Geometry check sheet. Reference: the model listing, model coordinates, mm. Face numbers are marked on the shaded views. A direction names the side the tool comes from. Round coordinates to 2 decimals unless told otherwise and drop trailing zeros. Write each loop counter-clockwise with the first axis right and the second up, starting at its lowest first coordinate (ties: lowest second). Pieces come first, ordered by that corner, then holes. Notation, with made-up numbers: (17, -17) -> (59, -17) arc R25 ccw to (59, 18) -> close; hole circle Ø9 at (20, -5.75). An arc over 180 degrees is marked (long way). Use a Markdown table: item, result.
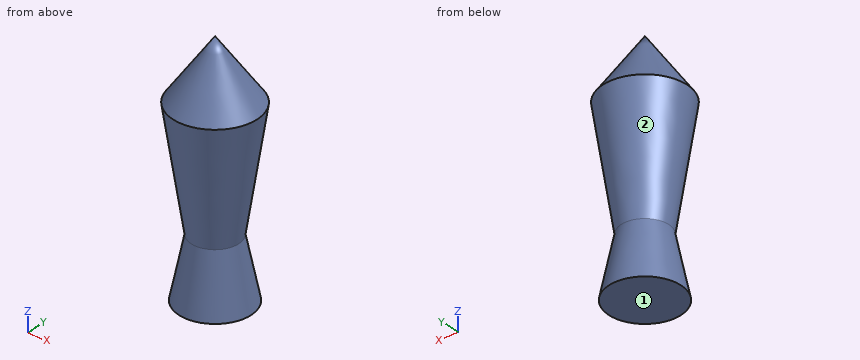
```python
from build123d import *


with BuildPart() as f1:
    # F0 (on Front) → F1 (revolve)
    with BuildSketch(Plane.XZ):
        Polygon((-15.24, 0), (0, 0), (0, 25.4), (-10.009029, 25.4), align=None)
    revolve(axis=Axis((0, 0, 12.7), (0, 0, -1)))

    # F2 (on Front) → F3 (revolve)
    with BuildSketch(Plane.XZ):
        Polygon((-17.78, 76.2), (-10.009029, 25.4), (0, 25.4), (0, 76.2), align=None)
    revolve(axis=Axis((0, 0, 50.8), (0, 0, 1)))

    # F4 (on Front) → F5 (revolve)
    with BuildSketch(Plane.XZ):
        Polygon((0, 101.6), (-17.78, 76.2), (0, 76.2), align=None)
    revolve(axis=Axis((0, 0, 88.9), (0, 0, 1)))


solid = f1.part
```
(1) Access from +Z, -Z, +X, -X, +Y, -Y to the whole of each face (thin tool, end or side, straight path). Record for the marked faces 1 and 2.
A:
| item | result |
|---|---|
| face 1 | -Z, +X, -X, +Y, -Y |
| face 2 | none |
(2) Section check B-B on z = 61.5. Record the cut outline in (x, y), plus the area to 3 significant figures.
A:
| item | result |
|---|---|
| outline | circle Ø31.06 at (0, 0) |
| area | 758 mm2 |
(3) Section check A-A on z = 79. Record the cut outline in (x, y).
A:
| item | result |
|---|---|
| outline | circle Ø31.64 at (0, 0) |
(4) Thickness scan on line 1 (X direction, y = -1, z = 97); line 2 (X direction, y = 3.5, z = 87.5); line 3 (Y direction, x = 2, z = 64). Record the ranges inside material, lowest first.
A:
| item | result |
|---|---|
| line 1 | x = -3.06 to 3.06 |
| line 2 | x = -9.23 to 9.23 |
| line 3 | y = -15.79 to 15.79 |
(5) Gauge pin test, flat ends, axial feed: pin 1 Ø2 at (x, z) = (-11.5, 62) entering from +Y; pin 2 Ø2 at (x, z) = (0.5, 75) entering from -Y; pin 3 Ø3 at (x, z) = (-6, 14) entering from -Y. Record the tip position at first contact, or that the pin passes through.
A:
| item | result |
|---|---|
| pin 1 | stops at y = 11.57 |
| pin 2 | stops at y = -17.74 |
| pin 3 | stops at y = -11.59 |
